Could you check a few things on this model? Use its own coordinates, in mm. Coordinates: 2 decimals unless noted, no trailing zeros. Order: outer loops, then holes, each group sorted by start corner. A loop starts at its lowest first (then second) coordinate and runs counter-clockwise, first axis right, second up. Notation, with made-up numbers: (43, 11) - (68, 11) arc R12 ccw to (68, 20) - close; hole circle Ø10 at (18, 42.5). An arc over 180 degrees is marked (long way). Answer as a JSON object with one key per item and string values. Group by question number.
(1) Will these pins go through, and if not, where does the flat tip stop? P1, Ø1.6, axis at x = 2, z = 2, coming from the -Y side; P2, Ø1.6, axis at y = 42.5, z = 1.5, coming from the +X side.
(2) Imagine slicing it at C-C, the plane x = -8.25. Write out the boundary of the cut face in (y, z) (3 decimals).
(3) Please list where these lines run through material, in increasing order: probe 1 along Y at (x, z) = (1.5, 2.45) (3 decimals); probe 2 along X at (y, z) = (33, 2.65); probe 3 along X at (y, z) = (58, 0.95).
(4) Imagine slicing it at B-B, the plane z = 1.55. Write out the boundary of the cut face in (x, y) (3 decimals).
(5) Imagine slicing it at A-A, the plane x = 1. Write out the boundary of the cut face in (y, z) (3 decimals), and give its area (3 significant figures).
(6) Imagine slicing it at D-D, the plane y = 79. Write out the boundary of the cut face in (x, z) (3 decimals).
from build123d import *

# Parameters (mm, degrees)
SKETCH1_W           = 3.175
SKETCH1_H           = 9.525
BOSS_EXTRUDE1_DEPTH = 3.175


with BuildPart() as part:
    # Sketch1 → Boss-Extrude1 (new body)
    with BuildSketch(Plane.XY):
        Polygon((0, 101.6), (-3.175, 101.6), (-25.4, 0), (0, 0), align=None)
        with Locations((1.5875, 68.2625)):
            Rectangle(SKETCH1_W, SKETCH1_H)
        with Locations((1.5875, 96.8375)):
            Rectangle(SKETCH1_W, SKETCH1_H)
    extrude(amount=BOSS_EXTRUDE1_DEPTH)


solid = part.part
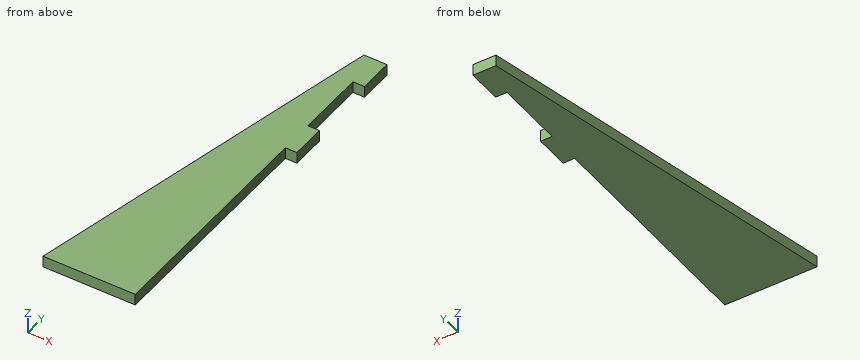
Result set:
{
 "1": {"P1": "stops at y = 63.5", "P2": "stops at x = 0"},
 "2": {"outline": "(0, 0) - (78.4, 0) - (78.4, 3.175) - (0, 3.175) - close"},
 "3": {"probe 1": "y = 63.5 to 73.025, 92.075 to 101.6", "probe 2": "x = -18.18 to 0", "probe 3": "x = -12.71 to 0"},
 "4": {"outline": "(-25.4, 0) - (0, 0) - (0, 63.5) - (3.175, 63.5) - (3.175, 73.025) - (0, 73.025) - (0, 92.075) - (3.175, 92.075) - (3.175, 101.6) - (-3.175, 101.6) - close"},
 "5": {"outline": "(63.5, 0) - (73.025, 0) - (73.025, 3.175) - (63.5, 3.175) - close; (92.075, 0) - (101.6, 0) - (101.6, 3.175) - (92.075, 3.175) - close", "area": "60.5 mm^2"},
 "6": {"outline": "(-8.119, 0) - (0, 0) - (0, 3.175) - (-8.119, 3.175) - close"}
}
